Source: CAD feature listing. Evaluate the final solid. Frame: model axes, mm. Face numbers are marked on the shaded views. A direction names the side the tool comes from. Round coordinates to 2 decimals unless told otherwise and drop trailing zeros. Order: outer loops, then holes, each group sorted by start corner. A loop starts at its lowest first (then second) coordinate and runs counter-clockwise, first axis right, second up. Notation, with made-up numbers: (84, -26.5) - (93, -26.5) arc R20 cw to (93, -7.5) - close; hole circle Ø11 at (67, 69). An arc over 180 degrees is marked (long way). Put each result on its own line as item: value. Start each with the question number.
1) Section B-B on x = -28.5. Output: boundary loops of the cut face in (y, z).
2) Section D-D on y = 13. Output: boundary loops of the cut face in (x, z).
3) Line query: probe 1 along Z at (x, y) = (-9.5, 8); probe 2 along Z at (x, y) = (-20, 15); probe 3 along Y at (x, z) = (-18, 44.5). Output: solid intervals per line, ascending. Write a range as [from, to].
4) Section C-C on y = 31. Output: boundary loops of the cut face in (x, z).
5) Contact query for flat-ended pins moving along their axis: P1, Ø4, axis at y = 9, z = 21, coming from the -X side; P2, Ø8, axis at x = -32.5, z = 14, coming from the -Y side (3 decimals); P3, Ø4, axis at x = -15, y = 5, coming from the -Z side; P4, Ø0.7, axis at x = -31, y = 26, coming from the -Z side. Output: stop coordinate, or through.
6) Access query for the marked faces 1, 2 and 3. Directions: +Z, -Z, +X, -X, +Y, -Y. A direction counts if a zero-diameter tool reaches every point of the face in a straight line with its end or side. Return the directions, or none.
7) Section A-A on z = 13. Output: boundary loops of the cut face in (x, y).
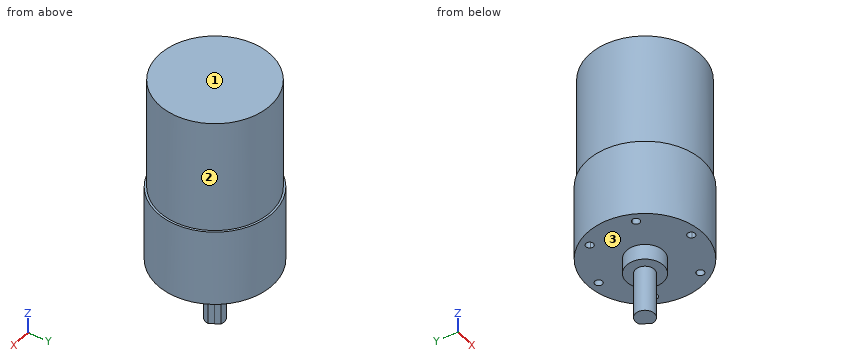
```python
from build123d import *

# Parameters (mm, degrees)
SKETCH2_R           = 18.499999957
BOSS_EXTRUDE1_DEPTH = 81
SKETCH3_R           = 34.5
SKETCH3_R_2         = 5.9
CUT_EXTRUDE1_DEPTH  = 20
SKETCH4_R           = 5.9
SKETCH4_R_2         = 3
CUT_EXTRUDE2_DEPTH  = 15
SKETCH6_R           = 34.5
SKETCH6_R_2         = 17.849200014
CUT_EXTRUDE3_DEPTH  = 36.4
CUT_EXTRUDE11_DEPTH = 15
CUT_EXTRUDE13_DEPTH = 25.4


with BuildPart() as part:
    # Sketch2 → Boss-Extrude1 (new body)
    with BuildSketch(Plane.XY):
        with Locations((-17.902568237, 17.753380168)):
            Circle(SKETCH2_R)
    extrude(amount=BOSS_EXTRUDE1_DEPTH)

    # Sketch3 → Cut-Extrude1 (cut)
    with BuildSketch(Plane(origin=(0, 0, 0), x_dir=(-1, 0, 0), z_dir=(0, 0, -1))):
        with Locations((17.902568237, 17.753380168)):
            Circle(SKETCH3_R)
        with Locations((17.902568237, 17.753380168)):
            Circle(SKETCH3_R_2, mode=Mode.SUBTRACT)
    extrude(amount=-CUT_EXTRUDE1_DEPTH, mode=Mode.SUBTRACT)

    # Sketch4 → Cut-Extrude2 (cut)
    with BuildSketch(Plane(origin=(0, 0, 0), x_dir=(-1, 0, 0), z_dir=(0, 0, -1))):
        with Locations((17.902568237, 17.753380168)):
            Circle(SKETCH4_R)
        with Locations((17.902568237, 17.753380168)):
            Circle(SKETCH4_R_2, mode=Mode.SUBTRACT)
    extrude(amount=-CUT_EXTRUDE2_DEPTH, mode=Mode.SUBTRACT)

    # Sketch6 → Cut-Extrude3 (cut)
    with BuildSketch(Plane.XY.offset(81)):
        with Locations((-17.902568237, 17.753380168)):
            Circle(SKETCH6_R)
        with Locations((-17.902568237, 17.753380168)):
            Circle(SKETCH6_R_2, mode=Mode.SUBTRACT)
    extrude(amount=-CUT_EXTRUDE3_DEPTH, mode=Mode.SUBTRACT)

    # Sketch12 → Cut-Extrude11 (cut)
    with BuildSketch(Plane(origin=(0, 0, 0), x_dir=(-1, 0, 0), z_dir=(0, 0, -1))):
        with BuildLine():
            Line((14.905470459, 17.621452506), (15.747198213, 19.020021419))
            Line((15.747198213, 19.020021419), (16.615935607, 20.463468077))
            ThreePointArc((16.615935607, 20.463468077), (15.33218895, 19.300361203), (14.905470459, 17.621452506))
        make_face()
    extrude(amount=-CUT_EXTRUDE11_DEPTH, mode=Mode.SUBTRACT)

    # Sketch13 → Cut-Extrude13 (cut)
    with BuildSketch(Plane(origin=(0, 0, 0), x_dir=(-1, 0, 0), z_dir=(0, 0, -1))):
        with BuildLine():
            ThreePointArc((5.152568237, 24.509673531), (5.099648896, 24.862102191), (4.945558303, 25.18344703))
            Line((4.945558303, 25.18344703), (3.952568237, 24.509673531))
            Line((3.952568237, 24.509673531), (4.039578171, 23.312832158))
            ThreePointArc((4.039578171, 23.312832158), (4.831320739, 23.692486869), (5.152568237, 24.509673531))
        make_face()
        with BuildLine():
            Line((3.952568237, 24.509673531), (4.945558303, 25.18344703))
            ThreePointArc((4.945558303, 25.18344703), (2.872568237, 25.032741404), (4.039578171, 23.312832158))
            Line((4.039578171, 23.312832158), (3.952568237, 24.509673531))
        make_face()
        with BuildLine():
            Line((17.858689924, 32.689513359), (16.778689924, 33.212581232))
            Line((16.778689924, 33.212581232), (15.785699858, 32.538807733))
            ThreePointArc((15.785699858, 32.538807733), (16.865699858, 32.01573986), (17.858689924, 32.689513359))
        make_face()
        with BuildLine():
            Line((15.785699858, 32.538807733), (16.778689924, 33.212581232))
            Line((16.778689924, 33.212581232), (17.858689924, 32.689513359))
            ThreePointArc((17.858689924, 32.689513359), (17.948305245, 32.944253075), (17.978689924, 33.212581232))
            ThreePointArc((17.978689924, 33.212581232), (16.426261264, 34.359661892), (15.785699858, 32.538807733))
        make_face()
        with BuildLine():
            ThreePointArc((6.276446549, 9.050472467), (5.893633211, 9.929224969), (4.989436616, 10.247313839))
            Line((4.989436616, 10.247313839), (5.076446549, 9.050472467))
            Line((5.076446549, 9.050472467), (6.156446549, 8.527404593))
            ThreePointArc((6.156446549, 8.527404593), (6.246061871, 8.782144309), (6.276446549, 9.050472467))
        make_face()
        with BuildLine():
            Line((5.076446549, 9.050472467), (4.989436616, 10.247313839))
            ThreePointArc((4.989436616, 10.247313839), (4.083456483, 8.376698967), (6.156446549, 8.527404593))
            Line((6.156446549, 8.527404593), (5.076446549, 9.050472467))
        make_face()
        with BuildLine():
            ThreePointArc((31.928689924, 26.45628787), (30.997018081, 27.625903191), (29.648689924, 26.979355743))
            Line((29.648689924, 26.979355743), (30.728689924, 26.45628787))
            Line((30.728689924, 26.45628787), (30.815699858, 25.259446497))
            ThreePointArc((30.815699858, 25.259446497), (31.607442426, 25.639101208), (31.928689924, 26.45628787))
        make_face()
        with BuildLine():
            Line((30.728689924, 26.45628787), (29.648689924, 26.979355743))
            ThreePointArc((29.648689924, 26.979355743), (29.735699858, 25.78251437), (30.815699858, 25.259446497))
            Line((30.815699858, 25.259446497), (30.728689924, 26.45628787))
        make_face()
        with BuildLine():
            ThreePointArc((33.052568237, 10.997086806), (32.669754898, 11.875839308), (31.765558303, 12.193928178))
            Line((31.765558303, 12.193928178), (31.852568237, 10.997086806))
            Line((31.852568237, 10.997086806), (30.859578171, 10.323313306))
            ThreePointArc((30.859578171, 10.323313306), (32.204996897, 9.850006146), (33.052568237, 10.997086806))
        make_face()
        with BuildLine():
            Line((31.852568237, 10.997086806), (31.765558303, 12.193928178))
            ThreePointArc((31.765558303, 12.193928178), (30.772568237, 11.520154679), (30.859578171, 10.323313306))
            Line((30.859578171, 10.323313306), (31.852568237, 10.997086806))
        make_face()
        with BuildLine():
            ThreePointArc((20.019436616, 2.967952604), (18.939436616, 3.491020477), (17.946446549, 2.817246977))
            Line((17.946446549, 2.817246977), (19.026446549, 2.294179104))
            Line((19.026446549, 2.294179104), (20.019436616, 2.967952604))
        make_face()
        with BuildLine():
            Line((19.026446549, 2.294179104), (17.946446549, 2.817246977))
            ThreePointArc((17.946446549, 2.817246977), (18.758118392, 1.124563783), (20.226446549, 2.294179104))
            ThreePointArc((20.226446549, 2.294179104), (20.173527209, 2.646607764), (20.019436616, 2.967952604))
            Line((20.019436616, 2.967952604), (19.026446549, 2.294179104))
        make_face()
    extrude(amount=-CUT_EXTRUDE13_DEPTH, mode=Mode.SUBTRACT)


solid = part.part
```
Answer sheet:
1. outline: (2.59, 20) - (32.92, 20) - (32.92, 44.6) - (32.12, 44.6) - (32.12, 81) - (3.39, 81) - (3.39, 44.6) - (2.59, 44.6) - close
2. outline: (-35.78, 20) - (-21.4, 20) - (-21.4, 15) - (-14.41, 15) - (-14.41, 20) - (-0.02, 20) - (-0.02, 44.6) - (-0.7, 44.6) - (-0.7, 81) - (-35.11, 81) - (-35.11, 44.6) - (-35.78, 44.6) - close
3. probe 1: [20, 81]
3. probe 2: [15, 81]
3. probe 3: [-0.75, 36.25]
4. outline: (-30.82, 20) - (-4.99, 20) - (-4.99, 44.6) - (-5.94, 44.6) - (-5.94, 81) - (-29.87, 81) - (-29.87, 44.6) - (-30.82, 44.6) - close
5. P1: x = -35.13
5. P2: through
5. P3: z = 20
5. P4: z = 25.4
6. face 1: +Z, +X, -X, +Y, -Y
6. face 2: +Z
6. face 3: -Z
7. outline: (-16.62, 20.46) arc R3 ccw (long way) to (-14.91, 17.62) - close
